```python
from build123d import *
from build123d import SkipClean  # not in build123d's __all__

# Parameters (mm, degrees)
F0_R     = 65.5
F1_DEPTH = 2
F2_R     = 65.5
F2_R_2   = 62.5
F3_DEPTH = 1


with BuildPart() as f1:
    # F0 (on Top) → F1 (new body)
    with BuildSketch(Plane.XY):
        Circle(F0_R)
        with BuildLine():
            ThreePointArc((32.9658290909, 53.0990029318), (54.1265877365, 31.25), (62.468, 1.9997439836))
            ThreePointArc((62.468, 1.9997439836), (64.5, 0), (62.468, -1.9997439836))
            ThreePointArc((62.468, -1.9997439836), (54.1265877365, -31.25), (32.9658290909, -53.0990029318))
            ThreePointArc((32.9658290909, -53.0990029318), (32.25, -55.8586385441), (29.5021709091, -55.0987469154))
            ThreePointArc((29.5021709091, -55.0987469154), (0, -62.5), (-29.5021709091, -55.0987469154))
            ThreePointArc((-29.5021709091, -55.0987469154), (-32.25, -55.8586385441), (-32.9658290909, -53.0990029318))
            ThreePointArc((-32.9658290909, -53.0990029318), (-54.1265877365, -31.25), (-62.468, -1.9997439836))
            ThreePointArc((-62.468, -1.9997439836), (-64.5, 0), (-62.468, 1.9997439836))
            ThreePointArc((-62.468, 1.9997439836), (-54.1265877365, 31.25), (-32.9658290909, 53.0990029318))
            ThreePointArc((-32.9658290909, 53.0990029318), (-32.25, 55.8586385441), (-29.5021709091, 55.0987469154))
            ThreePointArc((-29.5021709091, 55.0987469154), (0, 62.5), (29.5021709091, 55.0987469154))
            ThreePointArc((29.5021709091, 55.0987469154), (32.25, 55.8586385441), (32.9658290909, 53.0990029318))
        make_face(mode=Mode.SUBTRACT)
    extrude(amount=F1_DEPTH)

    # F2 (on Top) → F3 (join)
    with BuildSketch(Plane.XY):
        Circle(F2_R)
        Circle(F2_R_2, mode=Mode.SUBTRACT)
    with SkipClean():  # cleaning this boolean's faces spoils the solid; the shape is the same uncleaned
        extrude(amount=F3_DEPTH)


solid = f1.part
```
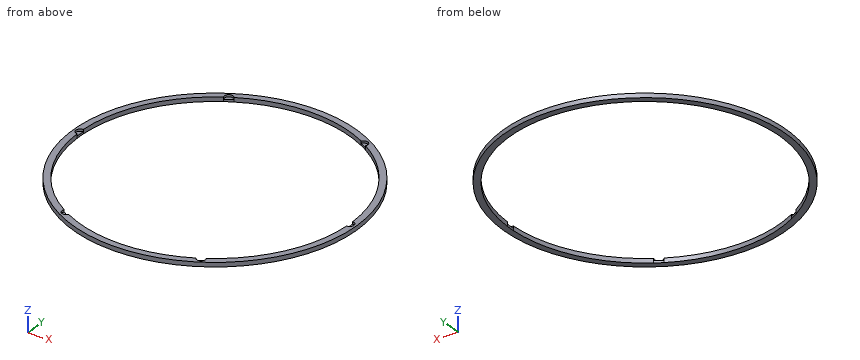
Here's how the part is built. I have some questions about the finished solid (model axes, mm). Give positions to 0.01 mm unless a question says otherwise; leave off trailing zeros. Order: outer loops, then holes, each group sorted by start corner. A loop starts at its lowest first (then second) coordinate and runs counter-clockwise, first axis right, second up. Notation, with made-up numbers: (-18.75, -20) - (3.25, -20) arc R29 ccw to (3.25, 17) - close; hole circle Ø7 at (19, -11.75). An arc over 180 degrees is marked (long way). Answer as a JSON object with one key per item and string values. Group by question number.
Item 1: If we section it at A-A on z = 1.7: Please give me the cut outline in (x, y), and give its area (3 significant figures).
Item 2: If we section it at B-B on x = 0: Please give me the cut outline in (y, z).
Item 3: If we section it at D-D on y = -29: Please give me the cut outline in (x, z).
Item 4: Please list where these lines run through material, in increasing order: probe 1 along X at (y, z) = (46, 0.65); probe 2 along Y at (x, z) = (37, 1.75); probe 3 along X at (y, z) = (22, 0.3).
Item 5: For P1, Ø3.5, axis at x = -31.5, y = -54.5, coming from the +Z side; P2, Ø0.9, axis at x = -31, y = 54.5, coming from the +Z side; P3, Ø1, axis at y = 16, z = 1, coming from the -X side; P4, Ø1, axis at x = -1, z = 1.5, coming from the -Y side, each with a flat end and sliding along its axis, tell me the tip position at first contact or that it passes through.
Item 6: If we section it at C-C on y = 0: Please give me the cut outline in (x, z), and give its area (3 significant figures).
Result set:
{
 "1": {"outline": "circle Ø131 at (0, 0); hole (-62.47, -2) arc R62.5 ccw to (-32.97, -53.1) arc R2 ccw (long way) to (-29.5, -55.1) arc R62.5 ccw to (29.5, -55.1) arc R2 ccw (long way) to (32.97, -53.1) arc R62.5 ccw to (62.47, -2) arc R2 ccw (long way) to (62.47, 2) arc R62.5 ccw to (32.97, 53.1) arc R2 ccw (long way) to (29.5, 55.1) arc R62.5 ccw to (-29.5, 55.1) arc R2 ccw (long way) to (-32.97, 53.1) arc R62.5 ccw to (-62.47, 2) arc R2 ccw (long way) to start", "area": "1,170 mm²"},
 "2": {"outline": "(-65.5, 0) - (-62.5, 0) - (-62.5, 2) - (-65.5, 2) - close; (62.5, 0) - (65.5, 0) - (65.5, 2) - (62.5, 2) - close"},
 "3": {"outline": "(-58.73, 0) - (-55.36, 0) - (-55.36, 2) - (-58.73, 2) - close; (55.36, 0) - (58.73, 0) - (58.73, 2) - (55.36, 2) - close"},
 "4": {"probe 1": "-46.63 to -42.31, 42.31 to 46.63", "probe 2": "-54.05 to -50.37, 50.37 to 54.05", "probe 3": "-61.69 to -58.5, 58.5 to 61.69"},
 "5": {"P1": "z = 2", "P2": "z = 1", "P3": "x = -63.64", "P4": "y = -65.5"},
 "6": {"outline": "(-65.5, 0) - (-62.5, 0) - (-62.5, 1) - (-64.5, 1) - (-64.5, 2) - (-65.5, 2) - close; (62.5, 0) - (65.5, 0) - (65.5, 2) - (64.5, 2) - (64.5, 1) - (62.5, 1) - close", "area": "8.00 mm²"}
}
